Check sheet for the modelled part. Datum: model origin and axes. Units: mm. Face numbers are marked on the shaded views. A direction names the side the tool comes from. Round coordinates to 2 decimals unless told otherwise and drop trailing zeros. Loops run counter-clockwise (first coordinate to the right, second up) from the corner with the lowest first, then second, coordinate; pieces in that order, holes last. Notation, with made-up numbers: (-4, -23.75) - (17, -23.75) arc R18 cw to (17, -18.75) - close; hole circle Ø6 at (71.25, -27.5). An arc over 180 degrees is marked (long way). Return JSON: item names as keys, results as strings.
Autodesk Inventor part; units mm, degrees
ref_plane "YZ Plane" through (0, 0, 0) normal (1, 0, 0) x (0, 1, 0)
ref_plane "XZ Plane" through (0, 0, 0) normal (0, 1, 0) x (-1, 0, 0)
ref_plane "XY Plane" through (0, 0, 0) normal (0, 0, 1) x (1, 0, 0)
sketch "Sketch1" plane through (0, 0, 0) normal (1, 0, 0) x (0, 1, 0)
  line L0 (0, 0) -> (2, 0)
  line L1 (2, 0) -> (2, -47.5)
  line L2 (2, -47.5) -> (0, -47.5)
  line L3 (0, -47.5) -> (0, 0)
  line L4 (0, 0) -> (41, 0)
  line L5 (41, 0) -> (41, -2)
  line L6 (41, -2) -> (0, -2)
  line L7 (0, -2) -> (0, 0)
  point P0 (2, -2)
  dimension "d0" = 2
  dimension "d1" = 47.5
  dimension "d2" = 41
  dimension "d3" = 2
extrude "Extrusion1" add sketch "Sketch1" along normal blind 40
sketch "Sketch2" plane through (0, 0, 0) normal (0, 0, 1) x (1, 0, 0)
  line L0 (20, 27.5) -> (20, 13.5) construction
  line L1 (13.5, 27.5) -> (13.5, 13.5)
  line L2 (26.5, 13.5) -> (26.5, 27.5)
  arc A0 (26.5, 27.5) -> (13.5, 27.5) centre (20, 27.5) ccw
  arc A1 (13.5, 13.5) -> (26.5, 13.5) centre (20, 13.5) ccw
  circle A2 centre (35, 20.5) radius 1.5
  circle A3 centre (27.5, 33.4904) radius 1.5
  circle A4 centre (12.5, 33.4904) radius 1.5
  circle A5 centre (5, 20.5) radius 1.5
  circle A6 centre (12.5, 7.5096) radius 1.5
  circle A7 centre (27.5, 7.5096) radius 1.5
  point P0 (0, 0)
  point P1 (20, 20.5)
  point P2 (20, 20.5)
  dimension "d6" = 14
  dimension "d7" = 13
  dimension "d8" = 3
  dimension "d11" = 360
extrude "Extrusion2" cut sketch "Sketch2" against normal blind 40
fillet "Fillet1" radius 20 2 edges at (40, 41, -1) (0, 41, -1)
sketch "Sketch3" plane through (0, 0, -47.5) normal (0, -1, 0) x (1, 0, 0)
  circle A0 centre (5, 40) radius 1.75
  line L0 (5, 40) -> (5, 7.5) construction
  line L1 (5, 40) -> (37.5, 40) construction
  line L2 (5, 7.5) -> (35, 7.5) construction
  circle A1 centre (5, 7.5) radius 1.75
  circle A2 centre (35, 40) radius 1.75
  circle A3 centre (35, 7.5) radius 1.75
  point P0 (0, 47.5)
  dimension "d16" = 3.5
  dimension "d17" = 32.5
  dimension "d18" = 90
  dimension "d19" = 30
  dimension "d20" = 90
  dimension "d23" = 32.5
  dimension "d26" = 30
extrude "Extrusion3" cut sketch "Sketch3" against normal blind 40
fillet "Fillet2" radius 5 2 edges at (40, 1, -47.5) (0, 1, -47.5)
sketch "Sketch4" plane through (0, 0, 0) normal (0, 0, 1) x (1, 0, 0)
  arc A0 (40, 21) -> (0, 21) centre (20, 21) ccw
  line L0 (0, 21) -> (0, 0)
  line L1 (0, 0) -> (40, 0)
  line L2 (40, 21) -> (40, 0)
  circle A1 centre (12.5, 33.4904) radius 1.5
  circle A2 centre (35, 20.5) radius 1.5
  circle A3 centre (27.5, 33.4904) radius 1.5
  circle A4 centre (5, 20.5) radius 1.5
  circle A5 centre (27.5, 7.5096) radius 1.5
  line L3 (26.5, 27.5) -> (26.5, 13.5)
  arc A6 (13.5, 13.5) -> (26.5, 13.5) centre (20, 13.5) ccw
  line L4 (13.5, 13.5) -> (13.5, 27.5)
  arc A7 (26.5, 27.5) -> (13.5, 27.5) centre (20, 27.5) ccw
  circle A8 centre (12.5, 7.5096) radius 1.5
  line L5 (35, 20.5) -> (5, 20.5) construction
  circle A9 centre (27.5, 33.4904) radius 1.875
  circle A10 centre (12.5, 33.4904) radius 1.875
  circle A11 centre (5, 20.5) radius 1.875
  circle A12 centre (12.5, 7.5096) radius 1.875
  circle A13 centre (27.5, 7.5096) radius 1.875
  circle A14 centre (35, 20.5) radius 1.875
  point P0 (20, 20.5)
  dimension "d58" = 3.75
  dimension "d61" = 360
extrude "Extrusion4" cut sketch "Sketch4" against normal blind 10 contours A9 | A10 | A11 | A12 | A13 | A14
sketch "Sketch5" plane through (0, 2, -2) normal (0, 1, 0) x (1, 0, 0)
  circle A0 centre (5, 38) radius 1.75
  circle A1 centre (5, 5.5) radius 1.75
  circle A2 centre (35, 38) radius 1.75
  circle A3 centre (35, 5.5) radius 1.75
  arc A4 (5, 45.5) -> (0, 40.5) centre (5, 40.5) ccw
  line L0 (0, 40.5) -> (0, 0)
  line L1 (0, 0) -> (40, 0)
  line L2 (40, 40.5) -> (40, 0)
  arc A5 (40, 40.5) -> (35, 45.5) centre (35, 40.5) ccw
  line L3 (5, 45.5) -> (35, 45.5)
  circle A6 centre (5, 38) radius 1.8
  circle A7 centre (5, 5.5) radius 1.8
  circle A8 centre (35, 38) radius 1.8
  circle A9 centre (35, 5.5) radius 1.8
  point P0 (0, -2)
  dimension "d47" = 0.05
  dimension "d50" = 32.5
  dimension "d53" = 30
extrude "Extrusion5" cut sketch "Sketch5" against normal blind 10 contours A6 | A7 | A8 | A9
sketch "Sketch8" plane through (0, 0, 0) normal (0, 0, 1) x (1, 0, 0)
  circle A0 centre (35, 20.5) radius 1.875
  circle A1 centre (5, 20.5) radius 1.875
  circle A2 centre (27.5, 33.4904) radius 1.875
  circle A3 centre (27.5, 7.5096) radius 1.875
  circle A4 centre (12.5, 7.5096) radius 1.875
  circle A5 centre (12.5, 33.4904) radius 1.875
  arc A6 (40, 21) -> (0, 21) centre (20, 21) ccw
  line L0 (0, 21) -> (0, 0)
  line L1 (0, 0) -> (40, 0)
  line L2 (40, 21) -> (40, 0)
  line L3 (26.5, 27.5) -> (26.5, 13.5)
  arc A7 (13.5, 13.5) -> (26.5, 13.5) centre (20, 13.5) ccw
  line L4 (13.5, 13.5) -> (13.5, 27.5)
  arc A8 (26.5, 27.5) -> (13.5, 27.5) centre (20, 27.5) ccw
extrude "Extrusion8" add sketch "Sketch8" along normal blind 1
sketch "Sketch9" plane through (5, 0, -47.5) normal (0, -1, 0) x (1, 0, 0)
  circle A0 centre (30, 7.5) radius 1.8
  circle A1 centre (0, 7.5) radius 1.8
  circle A2 centre (30, 40) radius 1.8
  circle A3 centre (0, 40) radius 1.8
  arc A4 (-5, 5) -> (0, 0) centre (0, 5) ccw
  line L0 (0, 0) -> (30, 0)
  arc A5 (30, 0) -> (35, 5) centre (30, 5) ccw
  line L1 (35, 5) -> (35, 48.5)
  line L2 (-5, 48.5) -> (35, 48.5)
  line L3 (-5, 5) -> (-5, 48.5)
  point P0 (-5, 47.5)
extrude "Extrusion9" add sketch "Sketch9" along normal blind 1
fillet "Fillet4" radius 1.5 8 edges at (0, 10, 1) (40, 10, 1) (20, 41, 1) (38.5355, -1, -46.0355) (20, -1, -47.5) (1.4645, -1, -46.0355) (0, -1, -20.75) (40, -1, -20.75)
fillet "Fillet5" radius 1 1 edges at (20, 2, -2)
properties part number "520 DC Gear Motor Bracket"
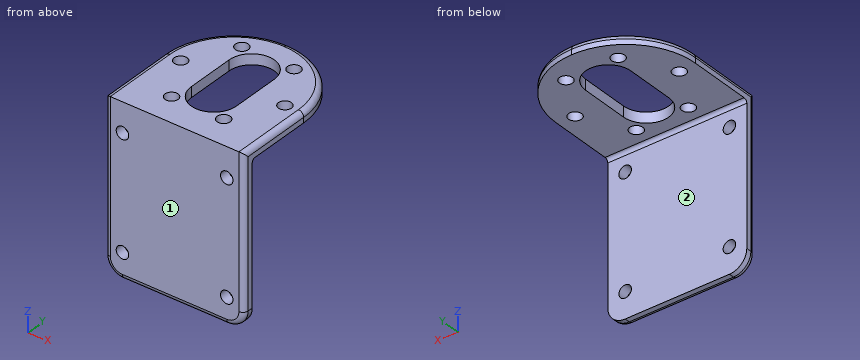
Q1. Sectioned sample at A-A (z = -7.5). Enter the section's corners in (x, y).
Answer key:
{"outline": "(0, 0.5) arc R1.5 ccw to (1.5, -1) - (3.2, -1) - (3.2, 2) - (0, 2) - close; (6.8, -1) - (33.2, -1) - (33.2, 2) - (6.8, 2) - close; (36.8, -1) - (38.5, -1) arc R1.5 ccw to (40, 0.5) - (40, 2) - (36.8, 2) - close"}
Q2. Tool access check on the marked faces 1 and 2. Record the directions out of +Z, -Z, +X, -X, +Y, -Y that give a thin tool (end or side, any length) a straight path to the whole face; none if there is none.
Answer key:
{"face 1": "+Z, -Z, +X, -X, -Y", "face 2": "-Z, +X, -X, +Y"}
Q3. Sectioned sample at B-B (z = -14). Enter the section's corners in (x, y), plus the area to 3 significant figures.
Answer key:
{"outline": "(0, 0.5) arc R1.5 ccw to (1.5, -1) - (38.5, -1) arc R1.5 ccw to (40, 0.5) - (40, 2) - (0, 2) - close", "area": "119 mm²"}
Q4. Depth check by flat-ended pin: P1, Ø20, axis at x = 25, z = -18.5, coming from the +Y side; P2, Ø11.5, axis at x = 16.5, y = 16, coming from the -Z side. Enter the tip coordinate at first touch or a pass-through.
Answer key:
{"P1": "stops at y = 2", "P2": "stops at z = -2"}
Q5. Sectioned sample at C-C (x = 28). State how many separate pieces and enclosed holes the cut face has, plus the area to 3 significant figures.
Answer key:
{"separate pieces": "3", "enclosed holes": "0", "area": "235 mm²"}
Q6. Scan lines: probe 1 along Z at (x, y) = (35, 0.45); probe 2 along Y at (x, z) = (27, 0); probe 3 along Y at (x, z) = (7, -21). Record each from-to range of solid material in increasing order. Write a range as [from, to].
Answer key:
{"probe 1": "z = [-47.5, -41.8], [-38.2, -9.3], [-5.7, 1]", "probe 2": "y = [-1, 5.7], [9.32, 31.68], [35.3, 39.64]", "probe 3": "y = [-1, 2]"}
